The drawing under review shows one solid part. Ordinate dimensions are in mm from its lowest x, y, z. Round coordinates to 2 decimals unless told otherwise and drop trailing zeros. Write each loop counter-clockwise with the first axis right and the second up, starting at its lowest first coordinate (ties: lowest second). Pieces come first, ordered by that corner, then holes. Notation, with made-up numbers: (22.25, 47.5) -> (64.25, 47.5) arc R17 ccw to (64.25, 56.5) -> close; hole circle Ø1 at (-17.75, 32). An arc over 180 degrees is marked (long way). Use CSV: the item, a comma, the result in double quotes. Start each with the question number.
1) For pin 1 Ø11 at (x, y) = (38, 60) entering from -Z; pin 2 Ø8 at (y, z) = (90.5, 4.5) entering from -X, all flat-tipped, find the tip position at first contact; note any pin that passes through.
2) Take a section at A-A, the plane y = 27. Give the boundary of the cut face in (x, z), then the cut area to 3 significant figures.
3) Mouldability with a two-part tool opening along X and no side actions: class the marked faces 1, 2, 3 and 4 as released by +X, released by -X, zero draft, split by the parting line, or undercut.
4) Take a section at C-C, the plane z = 1.5. Give the boundary of the cut face in (x, y), then the cut area to 3 significant figures.
5) Wall thickness on probe 1 along Y at (x, z) = (46, 10.5); probe 2 along Y at (x, z) = (43.5, 12); probe 3 along X at (y, z) = (96, 6.75): over which ranges is each line inside the solid? List them lowest first. Write a range as [from, to].
6) Take a section at D-D, the plane x = 36. Give the boundary of the cut face in (y, z), then the cut area to 3 significant figures.
7) Take a section at B-B, the plane x = 46. Give the boundary of the cut face in (y, z), then the cut area to 3 significant figures.
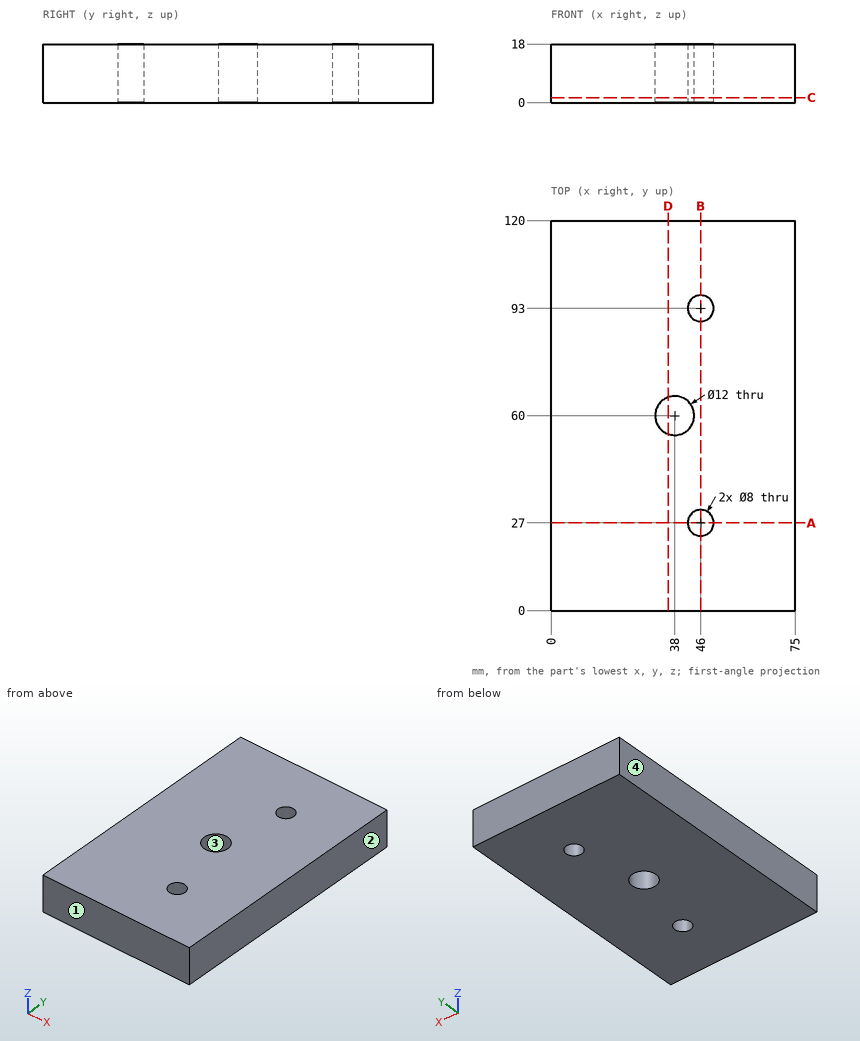
Values found:
1,pin 1,"through"
1,pin 2,"x = 0"
2,outline,"(0, 0) -> (42, 0) -> (42, 18) -> (0, 18) -> close; (50, 0) -> (75, 0) -> (75, 18) -> (50, 18) -> close"
2,area,"1,210 mm²"
3,face 1,"zero draft"
3,face 2,"released by +X"
3,face 3,"undercut"
3,face 4,"released by -X"
4,outline,"(0, 0) -> (75, 0) -> (75, 120) -> (0, 120) -> close; hole circle Ø12 at (38, 60); hole circle Ø8 at (46, 27); hole circle Ø8 at (46, 93)"
4,area,"8,790 mm²"
5,probe 1,"[0, 23], [31, 89], [97, 120]"
5,probe 2,"[0, 23.88], [30.12, 57.6], [62.4, 89.88], [96.12, 120]"
5,probe 3,"[0, 43.35], [48.65, 75]"
6,outline,"(0, 0) -> (54.34, 0) -> (54.34, 18) -> (0, 18) -> close; (65.66, 0) -> (120, 0) -> (120, 18) -> (65.66, 18) -> close"
6,area,"1,960 mm²"
7,outline,"(0, 0) -> (23, 0) -> (23, 18) -> (0, 18) -> close; (31, 0) -> (89, 0) -> (89, 18) -> (31, 18) -> close; (97, 0) -> (120, 0) -> (120, 18) -> (97, 18) -> close"
7,area,"1,870 mm²"
